Check sheet for the modelled part. Datum: model origin and axes. Units: mm. Face numbers are marked on the shaded views. A direction names the side the tool comes from. Round coordinates to 2 decimals unless told otherwise and drop trailing zeros. Write each loop counter-clockwise with the first axis right and the second up, starting at its lowest first coordinate (ties: lowest second). Pieces come first, ordered by that corner, then holes. Notation, with made-up numbers: M 72,-5.75 L 79,-5.75 A25 ccw 79,11.25 Z; hole C -23,59 d11. An arc over 180 degrees is marked long. Put each result on its own line as item: value.
```python
from build123d import *

# Parameters (mm, degrees)
F0_R      = 1.778
F1_DEPTH  = 15.24
F3_DEPTH  = 10.922
F4_R      = 5.08
F5_R      = 1.27
F6_R      = 2.794
F7_DEPTH  = 2.032
F9_DEPTH  = 1.6
F10_R     = 3
F11_DEPTH = 25
F12_R     = 3
F13_DEPTH = 25
F14_R     = 3
F15_DEPTH = 25
F16_R     = 3
F17_DEPTH = 25
F18_R     = 3
F19_DEPTH = 25


with BuildPart() as f1:
    # F0 (on Top) → F1 (new body)
    with BuildSketch(Plane.XY):
        Polygon((0, 56.7757548102), (0, 0), (34.544, 0), (34.544, 56.7757548102), (28.067, 70), (6.477, 70), align=None)
        with Locations((17.272, 4.953)):
            Circle(F0_R, mode=Mode.SUBTRACT)
        with Locations((17.272, 65.047)):
            Circle(F0_R, mode=Mode.SUBTRACT)
    extrude(amount=F1_DEPTH)

    # F2 (on face) → F3 (cut)
    with BuildSketch(Plane(origin=(0, 0, 0), x_dir=(1, 0, 0), z_dir=(0, 0, -1))):
        with BuildLine():
            Line((26.6411766499, -67.714), (32.258, -56.2459979667))
            Line((32.258, -56.2459979667), (32.258, -2.286))
            Line((32.258, -2.286), (22.987, -2.286))
            ThreePointArc((22.987, -2.286), (21.1011462146, -3.0671462146), (20.32, -4.953))
            ThreePointArc((20.32, -4.953), (17.272, -8.001), (14.224, -4.953))
            ThreePointArc((14.224, -4.953), (13.4428537854, -3.0671462146), (11.557, -2.286))
            Line((11.557, -2.286), (2.286, -2.286))
            Line((2.286, -2.286), (2.286, -56.2459979667))
            Line((2.286, -56.2459979667), (7.9028233501, -67.714))
            Line((7.9028233501, -67.714), (11.557, -67.714))
            ThreePointArc((11.557, -67.714), (13.4428537854, -66.9328537854), (14.224, -65.047))
            ThreePointArc((14.224, -65.047), (17.272, -61.999), (20.32, -65.047))
            ThreePointArc((20.32, -65.047), (21.1011462146, -66.9328537854), (22.987, -67.714))
            Line((22.987, -67.714), (26.6411766499, -67.714))
        make_face()
    extrude(amount=-F3_DEPTH, mode=Mode.SUBTRACT)

    # F4
    f4_edges = [f1.edges().sort_by_distance(p)[0] for p in [
        (6.477, 70, 7.62),
        (28.067, 70, 7.62),
        (34.544, 56.775755, 7.62),
        (34.544, 0, 7.62),
        (0, 0, 7.62),
        (0, 56.775755, 7.62),
    ]]
    fillet(f4_edges, radius=F4_R)

    # F5
    f5_edges = [f1.edges().sort_by_distance(p)[0] for p in [
        (1.487898, 1.487898, 15.24),
        (33.056102, 1.487898, 15.24),
        (34.412853, 56.745363, 15.24),
        (0.131147, 56.745363, 15.24),
        (27.586929, 69.23031, 15.24),
        (6.957071, 69.23031, 15.24),
        (17.272, 0, 15.24),
        (0, 30.339259, 15.24),
        (2.800565, 62.493735, 15.24),
        (17.272, 70, 15.24),
        (31.743435, 62.493735, 15.24),
        (34.544, 30.339259, 15.24),
    ]]
    fillet(f5_edges, radius=F5_R)

    # F6 (on face) → F7 (cut)
    with BuildSketch(Plane.XY.offset(15.24)):
        with Locations((17.272, 65.047)):
            Circle(F6_R)
        with Locations((17.272, 4.953)):
            Circle(F6_R)
    extrude(amount=-F7_DEPTH, mode=Mode.SUBTRACT)

    # F8 (on face) → F9 (cut)
    with BuildSketch(Plane.XY.offset(15.24)):
        Polygon((17.5, 18.4254264805), (12, 21.6008529611), (6.5, 18.4254264805), (6.5, 12.0745735195), (12, 8.8991470389), (17.5, 12.0745735195), align=None)
        Polygon((17.5, 38.4254264805), (12, 41.6008529611), (6.5, 38.4254264805), (6.5, 32.0745735195), (12, 28.8991470389), (17.5, 32.0745735195), align=None)
        Polygon((28.044, 42.0747205584), (28.044, 48.4255735195), (22.544, 51.601), (17.044, 48.4255735195), (17.044, 42.0747205584), (22.544, 38.8992940778), align=None)
        Polygon((6.5, 58.4254264805), (6.5, 52.0745735195), (12, 48.8991470389), (17.5, 52.0745735195), (17.5, 58.4254264805), (12, 61.6008529611), align=None)
        Polygon((28.044, 22.0747205584), (28.044, 28.4255735195), (22.544, 31.601), (17.044, 28.4255735195), (17.044, 22.0747205584), (22.544, 18.8992940778), align=None)
    extrude(amount=-F9_DEPTH, mode=Mode.SUBTRACT)

    # F10 (on face) → F11 (cut)
    with BuildSketch(Plane.XY.offset(13.64)):
        with Locations((12, 35.25)):
            Circle(F10_R)
    extrude(amount=-F11_DEPTH, mode=Mode.SUBTRACT)

    # F12 (on face) → F13 (cut)
    with BuildSketch(Plane.XY.offset(13.64)):
        with Locations((22.544, 45.2501470389)):
            Circle(F12_R)
    extrude(amount=-F13_DEPTH, mode=Mode.SUBTRACT)

    # F14 (on face) → F15 (cut)
    with BuildSketch(Plane.XY.offset(13.64)):
        with Locations((22.544, 25.2501470389)):
            Circle(F14_R)
    extrude(amount=-F15_DEPTH, mode=Mode.SUBTRACT)

    # F16 (on face) → F17 (cut)
    with BuildSketch(Plane.XY.offset(13.64)):
        with Locations((12, 15.25)):
            Circle(F16_R)
    extrude(amount=-F17_DEPTH, mode=Mode.SUBTRACT)

    # F18 (on face) → F19 (cut)
    with BuildSketch(Plane.XY.offset(13.64)):
        with Locations((12, 55.25)):
            Circle(F18_R)
    extrude(amount=-F19_DEPTH, mode=Mode.SUBTRACT)


solid = f1.part
```
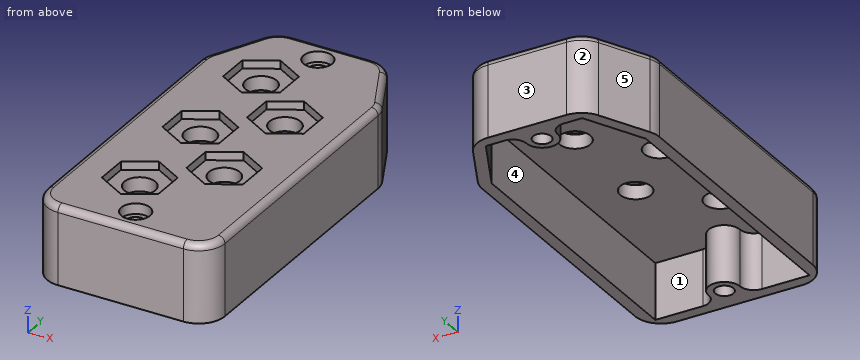
1. Scan lines: probe 1 along X at (y, z) = (7, 10.5); probe 2 along Y at (x, z) = (12, 13.25); probe 3 along Y at (x, z) = (23, 9.5). Record each from-to range of solid material in increasing order.
Computed values:
probe 1: x = 0 to 2.29, 15.01 to 19.53, 32.26 to 34.54
probe 2: y = 0 to 12.25, 18.25 to 32.25, 38.25 to 52.25, 58.25 to 70
probe 3: y = 0 to 2.29, 67.71 to 70
2. Cross-section at C-C (y = 30). Enter the section's corners in (x, z).
Computed values:
outline: M 0,0 L 2.29,0 L 2.29,10.92 L 32.26,10.92 L 32.26,0 L 34.54,0 L 34.54,13.97 A1.27 ccw 33.27,15.24 L 25.32,15.24 L 25.32,13.64 L 19.77,13.64 L 19.77,15.24 L 13.91,15.24 L 13.91,13.64 L 10.09,13.64 L 10.09,15.24 L 1.27,15.24 A1.27 ccw 0,13.97 Z
3. Cross-section at A-A (y = 15.25). Enter the section's corners in (x, z), then the cut area to 3 significant figures.
Computed values:
outline: M 0,0 L 2.29,0 L 2.29,10.92 L 9,10.92 L 9,13.64 L 6.5,13.64 L 6.5,15.24 L 1.27,15.24 A1.27 ccw 0,13.97 Z; M 15,10.92 L 32.26,10.92 L 32.26,0 L 34.54,0 L 34.54,13.97 A1.27 ccw 33.27,15.24 L 17.5,15.24 L 17.5,13.64 L 15,13.64 Z
area: 164 mm2
4. Release check for a two-part mould opening along X. For the marked faces 3, 4 and 5 record: +X half, -X half, draft (parallel to the pull), parting line (faces both ways), or undercut.
Computed values:
face 3: draft
face 4: undercut
face 5: -X half
5. Cross-section at B-B (z = 5). Enter the section's corners in (x, y), then the cut area to 3 significant figures.
Computed values:
outline: M 0,5.08 A5.08 ccw 5.08,0 L 29.46,0 A5.08 ccw 34.54,5.08 L 34.54,55.6 A5.08 ccw 34.03,57.83 L 29.46,67.15 A5.08 ccw 24.9,70 L 9.65,70 A5.08 ccw 5.08,67.15 L 0.52,57.83 A5.08 ccw 0,55.6 Z; hole M 2.29,2.29 L 11.56,2.29 A2.67 ccw 14.22,4.95 A3.05 cw 20.32,4.95 A2.67 ccw 22.99,2.29 L 32.26,2.29 L 32.26,56.25 L 26.64,67.71 L 22.99,67.71 A2.67 ccw 20.32,65.05 A3.05 cw 14.22,65.05 A2.67 ccw 11.56,67.71 L 7.9,67.71 L 2.29,56.25 Z; hole C 17.27,4.95 d3.56; hole C 17.27,65.05 d3.56
area: 469 mm2
6. Depth check by flat-ended pin: pin 1 Ø0.8 at (y, z) = (35.5, 14.5) entering from -X; pin 2 Ø5.5 at (x, y) = (22.54, 45.25) entering from +Z (1 decimal); pin 3 Ø9 at (x, y) = (11, 18) entering from +Z; pin 4 Ø9.5 at (x, y) = (12, 55.25) entering from -Z. Enter the tip coordinate at first touch or a pass-through.
Computed values:
pin 1: stops at x = 0.01
pin 2: passes through
pin 3: stops at z = 15.24
pin 4: stops at z = 10.92
7. Access from +Z, -Z, +X, -X, +Y, -Y to the whole of each face (thin tool, end or side, straight path). Record for the marked faces 1 and 2.
Computed values:
face 1: -Z
face 2: +Z, -Z, -X, +Y
